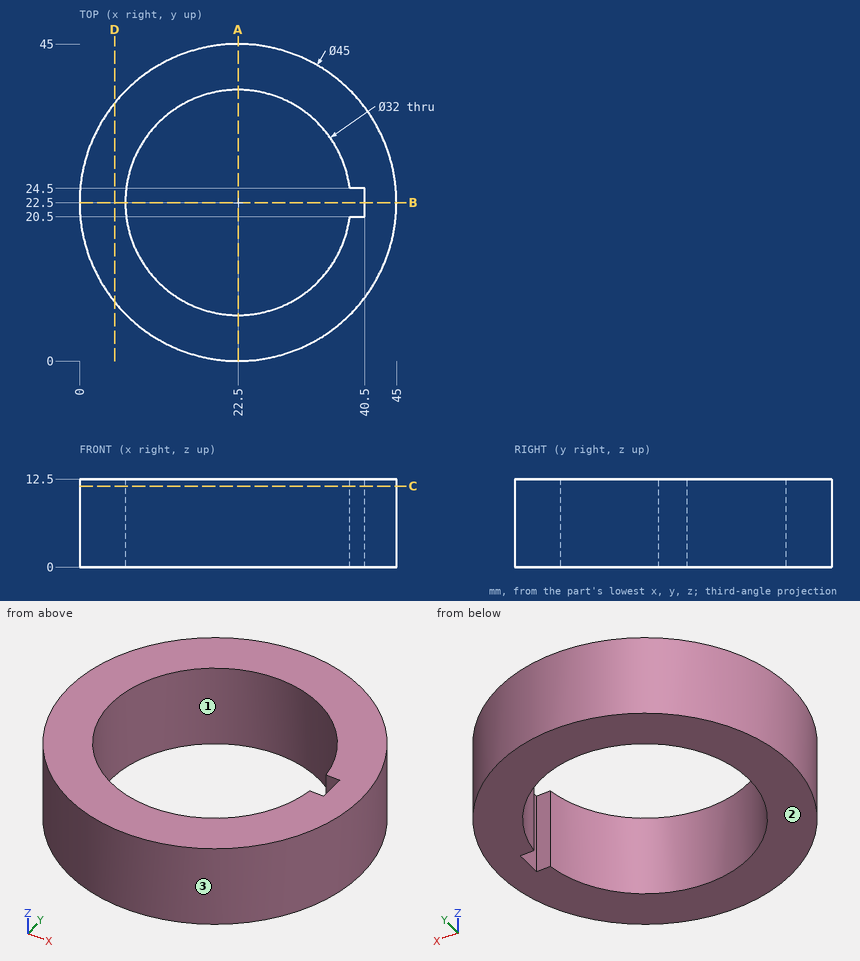
Study the drawing (mm; zero at the part's minimum x, y, z) and answer. Round coordinates to 2 decimals unless told otherwise and drop trailing zeros. Loops run counter-clockwise (first coordinate to the right, second up) from the corner with the lowest first, then second, coordinate; pieces in that order, holes last. Notation, with made-up numbers: (46.25, -19) -> (81.25, -19) arc R15 ccw to (81.25, 2) -> close; hole circle Ø10 at (28, 0). An arc over 180 degrees is marked (long way). One line per item, written item: value.
1) The mould has two halves that part along Y. Classify the marked faces 1, 2 and 3: pulls with the +Y half, pulls with the -Y half, needs draft (parallel to the pull), parting line crosses it, or undercut.
Answer list:
face 1: undercut
face 2: needs draft
face 3: parting line crosses it
2) Flat-ended cylindrical pins translate along their axes: P1, Ø6, axis at x = 38, y = 5, coming from the +Z side; P2, Ø6, axis at y = 27, z = 4, coming from the -X side; P3, Ø2.5, axis at x = 39.5, z = 6, coming from the -Y side; P4, Ø2.5, axis at x = 40, z = 4.5, coming from the +Y side. Find the tip coordinate at first contact, or state that the pin passes through.
Answer list:
P1: stops at z = 12.5
P2: stops at x = 0.05
P3: stops at y = 6.43
P4: stops at y = 38.06
3) A cutting plane is placed at C-C (z = 11.5). Determine the outline of the cut face in (x, y), and give its area (3 significant figures).
Answer list:
outline: circle Ø45 at (22.5, 22.5); hole (38.37, 20.5) -> (40.5, 20.5) -> (40.5, 24.5) -> (38.37, 24.5) arc R16 ccw (long way) to start
area: 778 mm²
4) Consider L1, parallel to Y at x = 22.5, z = 8; L2, parallel to Y at x = 14.5, z = 1; L3, parallel to X at y = 29, z = 3.5. Determine where each line is inside the solid, lowest interval first. Write a range as [from, to].
Answer list:
L1: y = [0, 6.5], [38.5, 45]
L2: y = [1.47, 8.64], [36.36, 43.53]
L3: x = [0.96, 7.88], [37.12, 44.04]
5) A cutting plane is placed at A-A (x = 22.5). Determine the outline of the cut face in (y, z).
Answer list:
outline: (0, 0) -> (6.5, 0) -> (6.5, 12.5) -> (0, 12.5) -> close; (38.5, 0) -> (45, 0) -> (45, 12.5) -> (38.5, 12.5) -> close
6) A cutting plane is placed at B-B (y = 22.5). Determine the outline of the cut face in (x, z).
Answer list:
outline: (0, 0) -> (6.5, 0) -> (6.5, 12.5) -> (0, 12.5) -> close; (40.5, 0) -> (45, 0) -> (45, 12.5) -> (40.5, 12.5) -> close
7) A cutting plane is placed at D-D (x = 5). Determine the outline of the cut face in (y, z).
Answer list:
outline: (8.36, 0) -> (36.64, 0) -> (36.64, 12.5) -> (8.36, 12.5) -> close
